from build123d import *

# Parameters (mm, degrees)
F0_R     = 33
F1_DEPTH = 6
F2_R     = 28.763366
F3_DEPTH = 2
F4_R     = 14.9859
F5_DEPTH = 2
F6_R     = 6.84366
F7_DEPTH = 4
F8_R     = 1.5
F9_DEPTH = 25


with BuildPart() as f1:
    # F0 (on Front) → F1 (new body)
    with BuildSketch(Plane.XZ):
        Circle(F0_R)
    extrude(amount=F1_DEPTH)

    # F2 (on face) → F3 (cut)
    with BuildSketch(Plane.XZ.offset(6)):
        Circle(F2_R)
    extrude(amount=-F3_DEPTH, mode=Mode.SUBTRACT)

    # F4 (on face) → F5 (join)
    with BuildSketch(Plane.XZ.offset(4)):
        Circle(F4_R)
    extrude(amount=F5_DEPTH)

    # F6 (on face) → F7 (join)
    with BuildSketch(Plane.XZ.offset(6)):
        Circle(F6_R)
    extrude(amount=F7_DEPTH)

    # F8 (on face) → F9 (cut)
    with BuildSketch(Plane.XZ.offset(10)):
        Circle(F8_R)
    extrude(amount=-F9_DEPTH, mode=Mode.SUBTRACT)


solid = f1.part
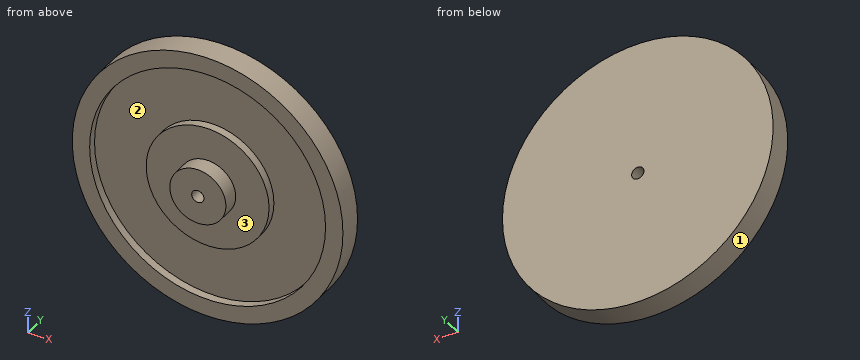
Input: part model. Units: mm. Frame: model coordinates. Face numbers are marked on the shaded views. Give positions to 0.01 mm unless a question says otherwise; leave off trailing zeros. Write each loop counter-clockwise with the first axis right and the second up, starting at its lowest first coordinate (ties: lowest second). Pieces come first, ordered by that corner, then holes. Notation, with made-up numbers: (-37.75, 85.25) -> (-11.75, 85.25) arc R26 cw to (-11.75, 107.25) -> close; hole circle Ø2 at (34.5, 10.5). An arc over 180 degrees is marked (long way). Use one line per item in the form item = value. Start each with the question number.
1) Ray query, probe 1 along Z at (x, y) = (0, -9); probe 2 along Z at (x, y) = (0, -2.75); probe 3 along X at (y, z) = (-5.25, 13). Return the intervals inside material, ascending. Write a range as from..to.
2) Section query A-A on z = 0. Return the cut outline in (x, y).
3) Pin query (flat end, axial travel): pin 1 (5 mm diameter, centred on y = -4.5, z = 4.5, fed in from +X); pin 2 (3 mm diameter, centred on x = 7.5, z = 25, fed in from -Y); pin 3 (17.5 mm diameter, centred on x = 12.5, z = 12.5, fed in from -Y); pin 4 (1 mm diameter, centred on y = -8.5, z = 8, fed in from +X). Return the tip coordinate at first contact, or that it passes through.
4) Section query D-D on x = -12.5. Return the cut outline in (y, z), then the cut area to 3 significant figures.
5) Section query B-B on x = 0. Return the cut outline in (y, z).
6) Section query C-C on y = -8. Return the cut outline in (x, z).
7) Draft query along Z for the marked faces 1, 2 and 3. Return one class per face: pulls with the +Z half, pulls with the -Z half, needs draft (parallel to the pull), parting line crosses it, or undercut.
Outcome:
q1.probe_1 = -6.84..-1.5, 1.5..6.84
q1.probe_2 = -33..-1.5, 1.5..33
q1.probe_3 = -30.33..-25.66, -7.46..7.46, 25.66..30.33
q2.outline = (-33, -6) -> (-28.76, -6) -> (-28.76, -4) -> (-14.99, -4) -> (-14.99, -6) -> (-6.84, -6) -> (-6.84, -10) -> (-1.5, -10) -> (-1.5, 0) -> (-33, 0) -> close; (1.5, -10) -> (6.84, -10) -> (6.84, -6) -> (14.99, -6) -> (14.99, -4) -> (28.76, -4) -> (28.76, -6) -> (33, -6) -> (33, 0) -> (1.5, 0) -> close
q3.pin_1 = 32.94
q3.pin_2 = -4
q3.pin_3 = -6
q3.pin_4 = through
q4.outline = (-6, -30.54) -> (0, -30.54) -> (0, 30.54) -> (-6, 30.54) -> (-6, 25.91) -> (-4, 25.91) -> (-4, 8.27) -> (-6, 8.27) -> (-6, -8.27) -> (-4, -8.27) -> (-4, -25.91) -> (-6, -25.91) -> close
q4.area = 296 mm^2
q5.outline = (-10, -6.84) -> (-6, -6.84) -> (-6, -14.99) -> (-4, -14.99) -> (-4, -28.76) -> (-6, -28.76) -> (-6, -33) -> (0, -33) -> (0, -1.5) -> (-10, -1.5) -> close; (-10, 1.5) -> (0, 1.5) -> (0, 33) -> (-6, 33) -> (-6, 28.76) -> (-4, 28.76) -> (-4, 14.99) -> (-6, 14.99) -> (-6, 6.84) -> (-10, 6.84) -> close
q6.outline = circle Ø13.69 at (0, 0); hole circle Ø3 at (0, 0)
q7.face_1 = parting line crosses it
q7.face_2 = undercut
q7.face_3 = needs draft
